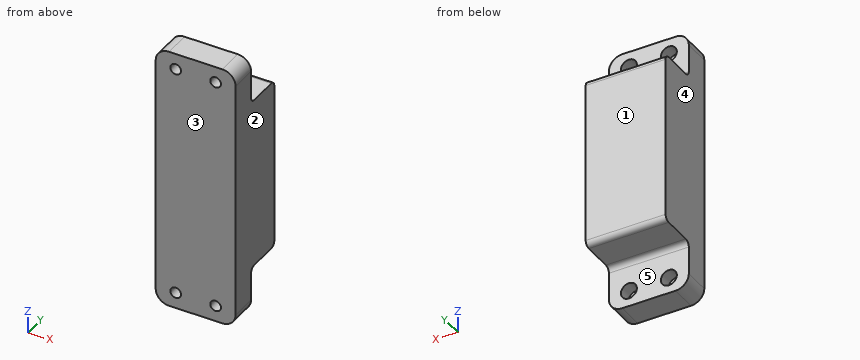
```python
from build123d import *

# Parameters (mm, degrees)
BOSS_EXTRUDE1_DEPTH                      = 30
FILLET1_R                                = 10
CBORE_FOR_M12_HEX_HEAD_BOLT1_D           = 8
CBORE_FOR_M12_HEX_HEAD_BOLT1_CBORE_D     = 12
CBORE_FOR_M12_HEX_HEAD_BOLT1_CBORE_DEPTH = 10


with BuildPart() as part:
    # Sketch1 → Boss-Extrude1 (new, symmetric)
    with BuildSketch(Plane(origin=(0, 0, 0), x_dir=(0, 0, -1), z_dir=(1, 0, 0))):
        with BuildLine():
            Line((100, 0), (-100, 0))
            Line((-100, 0), (-100, 20))
            Line((-100, 20), (-69, 20))
            ThreePointArc((-69, 20), (-66.171572875, 21.171572875), (-65, 24))
            Line((-65, 24), (-65, 46))
            ThreePointArc((-65, 46), (-63.828427125, 48.828427125), (-61, 50))
            Line((-61, 50), (61, 50))
            ThreePointArc((61, 50), (63.828427125, 48.828427125), (65, 46))
            Line((65, 46), (65, 24))
            ThreePointArc((65, 24), (66.171572875, 21.171572875), (69, 20))
            Line((69, 20), (100, 20))
            Line((100, 20), (100, 0))
        make_face()
    extrude(amount=BOSS_EXTRUDE1_DEPTH, both=True)

    # Fillet1
    fillet1_edges = [part.edges().sort_by_distance(p)[0] for p in [
        (-30, 10, 100),
        (-30, 10, -100),
        (30, 10, 100),
        (30, 10, -100),
    ]]
    fillet(fillet1_edges, radius=FILLET1_R)

    # CBORE for M12 Hex Head Bolt1 (through all)
    with Locations(Plane(origin=(0, 20, 0), x_dir=(1, 0, 0), z_dir=(0, 1, 0))):
        with Locations((-15, -88), (15, -88), (15, 88), (-15, 88)):
            CounterBoreHole(CBORE_FOR_M12_HEX_HEAD_BOLT1_D / 2, CBORE_FOR_M12_HEX_HEAD_BOLT1_CBORE_D / 2, CBORE_FOR_M12_HEX_HEAD_BOLT1_CBORE_DEPTH)


solid = part.part
```
Here's how the part is built. I have some questions about the finished solid (model axes, mm). Face numbers are marked on the shaded views. A direction names the side the tool comes from. Round coordinates to 2 decimals unless told otherwise and drop trailing zeros. Loops run counter-clockwise (first coordinate to the right, second up) from the corner with the lowest first, then second, coordinate; pieces in that order, holes last.
1. If I drill on probe 1 along X at (y, z) = (17, -88); probe 2 along Z at (x, y) = (-15, 4); probe 3 along Z at (x, y) = (-15, 12.25), over which ranges is the centre line in solid material (lowest first)?
Answers:
probe 1: x = -30 to -21, -9 to 9, 21 to 30
probe 2: z = -100 to -92, -84 to 84, 92 to 100
probe 3: z = -100 to -94, -82 to 82, 94 to 100
2. Suppose I cut it at A-A, the plane x = -15. Please give me the cut outline in (y, z).
Answers:
outline: (0, -100) - (20, -100) - (20, -94) - (10, -94) - (10, -92) - (0, -92) - close; (0, -84) - (10, -84) - (10, -82) - (20, -82) - (20, -69) arc R4 cw to (24, -65) - (46, -65) arc R4 ccw to (50, -61) - (50, 61) arc R4 ccw to (46, 65) - (24, 65) arc R4 cw to (20, 69) - (20, 82) - (10, 82) - (10, 84) - (0, 84) - close; (0, 92) - (10, 92) - (10, 94) - (20, 94) - (20, 100) - (0, 100) - close
3. Suppose I cut it at B-B, the plane y = 15. Please give me the cut outline in (x, z).
Answers:
outline: (-30, -90) arc R10 ccw to (-20, -100) - (20, -100) arc R10 ccw to (30, -90) - (30, 90) arc R10 ccw to (20, 100) - (-20, 100) arc R10 ccw to (-30, 90) - close; hole circle Ø12 at (-15, -88); hole circle Ø12 at (-15, 88); hole circle Ø12 at (15, -88); hole circle Ø12 at (15, 88)
4. Thinking about a two-plate mould opening in Y: for the marked faces 1, 2 and 3, which applies, released by +Y, released by -Y, zero draft, split by the parting line, or undercut?
Answers:
face 1: released by +Y
face 2: zero draft
face 3: released by -Y
5. Suppose I cut it at C-C, the plane z = 88. Please give me the cut outline in (x, y), and give its area (3 significant figures).
Answers:
outline: (-30, 0) - (-19, 0) - (-19, 10) - (-21, 10) - (-21, 20) - (-30, 20) - close; (-11, 0) - (11, 0) - (11, 10) - (9, 10) - (9, 20) - (-9, 20) - (-9, 10) - (-11, 10) - close; (19, 0) - (30, 0) - (30, 20) - (21, 20) - (21, 10) - (19, 10) - close
area: 800 mm2
6. Will these pins go through, and if not, where does the flat tip stop? pin 1 (6.5 mm diameter, centred on x = 15, z = 88, fed in from +Y); pin 2 (9.5 mm diameter, centred on x = 16, z = -88, fed in from +Y); pin 3 (24 mm diameter, centred on x = -7, y = 40, fed in from +Z); pin 4 (13 mm diameter, centred on x = -13.5, z = 86.5, fed in from +Y).
Answers:
pin 1: passes through
pin 2: stops at y = 10
pin 3: stops at z = 65
pin 4: stops at y = 20
7. Suppose I cut it at D-D, the plane x = -24. Please give me the cut outline in (y, z), and give its area (3 significant figures).
Answers:
outline: (0, -99.17) - (20, -99.17) - (20, -69) arc R4 cw to (24, -65) - (46, -65) arc R4 ccw to (50, -61) - (50, 61) arc R4 ccw to (46, 65) - (24, 65) arc R4 cw to (20, 69) - (20, 99.17) - (0, 99.17) - close
area: 7,870 mm2
8. For the marked faces 4 and 5, which set-ups out of +Z, -Z, +X, -X, +Y, -Y let a thin tool reach every point of the face, with its end or its side?
Answers:
face 4: +Z, -Z, -X, +Y, -Y
face 5: -Z, +X, -X, +Y
